```python
from build123d import *

# Parameters (mm, degrees)
F0_W     = 50
F0_H     = 12
F0_R     = 2.9335
F1_DEPTH = 5
F2_W     = 18.531616
F2_H     = 12
F2_W_2   = 18.120926
F3_DEPTH = 9
F4_R     = 2.9335
F5_DEPTH = 25
F6_W     = 50
F6_H     = 12
F7_DEPTH = 1


with BuildPart() as f1:
    # F0 (on Front) → F1 (new body)
    with BuildSketch(Plane.XZ):
        Rectangle(F0_W, F0_H)
        with Locations((-14, 0)):
            Circle(F0_R, mode=Mode.SUBTRACT)
        with Locations((14, 0)):
            Circle(F0_R, mode=Mode.SUBTRACT)
    extrude(amount=F1_DEPTH)

    # F2 (on face) → F3 (join)
    with BuildSketch(Plane.XZ.offset(5)):
        with Locations((-15.734192, 0)):
            Rectangle(F2_W, F2_H)
        with Locations((15.939537, 0)):
            Rectangle(F2_W_2, F2_H)
    extrude(amount=F3_DEPTH)

    # F4 (on face) → F5 (cut)
    with BuildSketch(Plane(origin=(0, 0, 0), x_dir=(-1, 0, 0), z_dir=(0, 1, 0))):
        with Locations((-14, 0)):
            Circle(F4_R)
        with Locations((14, 0)):
            Circle(F4_R)
    extrude(amount=-F5_DEPTH, mode=Mode.SUBTRACT)

    # F6 (on face) → F7 (join)
    with BuildSketch(Plane(origin=(0, 0, 0), x_dir=(-1, 0, 0), z_dir=(0, 1, 0))):
        Rectangle(F6_W, F6_H)
    extrude(amount=F7_DEPTH)


solid = f1.part
```
CAD build for the part. Positions are in the model's coordinates, mm. A direction names the side the tool comes from. Round coordinates to 2 decimals unless told otherwise and drop trailing zeros. Order: outer loops, then holes, each group sorted by start corner. A loop starts at its lowest first (then second) coordinate and runs counter-clockwise, first axis right, second up. Notation, with made-up numbers: (-28, 71) - (7, 71) arc R29 cw to (7, 110) - close; hole circle Ø5 at (-37, 44.5). An arc over 180 degrees is marked (long way). Answer in a Markdown table with one row per item. Add a question column.
(1) 3-axis set-ups, long thin cutter, end or side, ignore diameter. For faces 5 (the face through (0, -5, 0)), 6 (the face through (-25, -7, 0)): which of +Z, -Z, +X, -X, +Y, -Y reach the whole face in a straight line?
(2) Band-saw the part on C-C on x = -14. List the corners of the cut face in (y, z), and give its area (3 significant figures).
(3) Probe L1, parallel to X at y = -8.75, z = 0; L2, parallel to Z at x = 14, y = -8; L3, parallel to X at y = -8, z = -4.75. List the from-to ranges inside material, lowest first. Write a range as [from, to].
(4) Band-saw the part on B-B on y = -4.25. List the corners of the cut face in (x, z).
(5) Band-saw the part on A-A on y = -7. List the corners of the cut face in (x, z).
(6) Band-saw the part on D-D on z = 3.75. List the corners of the cut face in (x, y).
(7) Drop flat-ended pins along their axis: pin 1 Ø4.5 at (x, z) = (-14, 0) entering from -Y; pin 2 Ø4.5 at (x, z) = (-15, 0) entering from -Y; pin 3 Ø6 at (x, z) = (-1, -1.5) entering from -Y. Give the stop position or say it passes through.
(8) Mould opens along Z. For faces 1 (the face through (14, 0, 0)), 2 (the face through (-18, -14, 0)), 3 (the face through (-14, 0, 0)), 4 (the face through (0, -3, -6)) say: +Z half, -Z half, draft (parallel to the pull), parting line (faces both ways), or undercut.
Data:
| question | item | result |
|---|---|---|
| 1 | face 5 | +Z, -Z, -Y |
| 1 | face 6 | +Z, -Z, -X, +Y, -Y |
| 2 | outline | (-14, -6) - (1, -6) - (1, 6) - (-14, 6) - (-14, 2.93) - (0, 2.93) - (0, -2.93) - (-14, -2.93) - close |
| 2 | area | 97.9 mm^2 |
| 3 | L1 | x = [-25, -16.93], [-11.07, -6.47], [6.88, 11.07], [16.93, 25] |
| 3 | L2 | z = [-6, -2.93], [2.93, 6] |
| 3 | L3 | x = [-25, -6.47], [6.88, 25] |
| 4 | outline | (-25, -6) - (25, -6) - (25, 6) - (-25, 6) - close; hole circle Ø5.87 at (-14, 0); hole circle Ø5.87 at (14, 0) |
| 5 | outline | (-25, -6) - (-6.47, -6) - (-6.47, 6) - (-25, 6) - close; (6.88, -6) - (25, -6) - (25, 6) - (6.88, 6) - close; hole circle Ø5.87 at (-14, 0); hole circle Ø5.87 at (14, 0) |
| 6 | outline | (-25, -14) - (-6.47, -14) - (-6.47, -5) - (6.88, -5) - (6.88, -14) - (25, -14) - (25, 1) - (-25, 1) - close |
| 7 | pin 1 | stops at y = 0 |
| 7 | pin 2 | stops at y = -14 |
| 7 | pin 3 | stops at y = -5 |
| 8 | face 1 | undercut |
| 8 | face 2 | draft |
| 8 | face 3 | undercut |
| 8 | face 4 | -Z half |
